```python
from build123d import *

# Parameters (mm, degrees)
SKETCH_1_W          = 30
SKETCH_1_H          = 30
EXTRUDE_1_DEPTH     = 7
SKETCH_2_W          = 8.25
SKETCH_2_H          = 8.25
CUT_EXTRUDE_1_DEPTH = 23.338307904
SKETCH_3_R          = 3
EXTRUDE_2_DEPTH     = 2
SKETCH_4_R          = 1.6
CUT_EXTRUDE_2_DEPTH = 5
SKETCH_5_R          = 12.625
CUT_EXTRUDE_3_DEPTH = 3
FILLET_1_R          = 15


with BuildPart() as part:
    # Эскиз1 → Бобышка-Вытянуть1 (new body)
    with BuildSketch(Plane.XY):
        Rectangle(SKETCH_1_W, SKETCH_1_H)
    extrude(amount=EXTRUDE_1_DEPTH)

    # Эскиз2 → Вырез-Вытянуть1 (cut, through all)
    with BuildSketch(Plane.XY.offset(7)):
        Rectangle(SKETCH_2_W, SKETCH_2_H)
    extrude(amount=-CUT_EXTRUDE_1_DEPTH, mode=Mode.SUBTRACT)

    # Эскиз3 → Бобышка-Вытянуть2 (add)
    with BuildSketch(Plane.XY.offset(7)):
        with Locations((11.5, 0)):
            Circle(SKETCH_3_R)
        with Locations(Location((-11.5, 0, 0), (0, 0, 180))):
            Circle(SKETCH_3_R)
    extrude(amount=EXTRUDE_2_DEPTH)

    # Эскиз4 → Вырез-Вытянуть2 (cut)
    with BuildSketch(Plane.XY.offset(9)):
        with Locations((-11.5, 0)):
            Circle(SKETCH_4_R)
        with Locations((11.5, 0)):
            Circle(SKETCH_4_R)
    extrude(amount=-CUT_EXTRUDE_2_DEPTH, mode=Mode.SUBTRACT)

    # Эскиз5 → Вырез-Вытянуть3 (cut)
    with BuildSketch(Plane(origin=(0, 0, 0), x_dir=(-1, 0, 0), z_dir=(0, 0, -1))):
        Circle(SKETCH_5_R)
    extrude(amount=-CUT_EXTRUDE_3_DEPTH, mode=Mode.SUBTRACT)

    # Скругление1
    fillet_1_edges = [part.edges().sort_by_distance(p)[0] for p in [
        (-15, 15, 3.5),
        (15, 15, 3.5),
        (15, -15, 3.5),
        (-15, -15, 3.5),
    ]]
    fillet(fillet_1_edges, radius=FILLET_1_R - 0.0001)  # a hair under: the kernel refuses the full size


solid = part.part
```
Geometry check sheet. Reference: the model listing, model coordinates, mm. A direction names the side the tool comes from. Coordinates: 2 decimals unless noted, no trailing zeros. Order: outer loops, then holes, each group sorted by start corner. A loop starts at its lowest first (then second) coordinate and runs counter-clockwise, first axis right, second up.
Q1. Depth check by flat-ended pin: pin 1 Ø1 at (x, y) = (10.5, -4) entering from -Z; pin 2 Ø1 at (y, z) = (-7.5, 2) entering from +X; pin 3 Ø1 at (x, z) = (6, 1.5) entering from +Y. Enter the tip coordinate at first touch or a pass-through.
Reply:
pin 1: stops at z = 3
pin 2: stops at x = 13.27
pin 3: stops at y = 13.96
Q2. Sectioned sample at D-D on x = 9.5. Record the cut outline in (y, z), and give its area (3 significant figures).
Reply:
outline: (-11.61, 0) - (-8.32, 0) - (-8.32, 3) - (8.32, 3) - (8.32, 0) - (11.61, 0) - (11.61, 7) - (2.24, 7) - (2.24, 9) - (-2.24, 9) - (-2.24, 7) - (-11.61, 7) - close
area: 122 mm2
Q3. Tool access check on faces 1 (the face through (0, 4.125, 5)), 2 (the face through (-10.72, 10.49, 3.55)), 3 (the face through (0, -5, 3)), 4 (the face through (-12, 0, 4)), 5 (the face through (10.49, -10.72, 3.55)). Record the directions out of +Z, -Z, +X, -X, +Y, -Y that give a thin tool (end or side, any length) a straight path to the whole face; none if there is none.
Reply:
face 1: +Z, -Z
face 2: +Z, -Z, -X, +Y
face 3: -Z
face 4: +Z
face 5: +Z, -Z, +X, -Y
Q4. Thickness scan on probe 1 along Y at (x, z) = (0, 2.2) (3 decimals); probe 2 along Z at (x, y) = (2, -4.5); probe 3 along X at (y, z) = (-2, 1). Record the ranges inside material, lowest first.
Reply:
probe 1: y = -15 to -12.625, 12.625 to 15
probe 2: z = 3 to 7
probe 3: x = -14.87 to -12.47, 12.47 to 14.87
Q5. Sectioned sample at B-B on z = 8.25. Record the cut outline in (x, y), and give its area (3 significant figures).
Reply:
outline: circle Ø6 at (-11.5, 0); circle Ø6 at (11.5, 0); hole circle Ø3.2 at (-11.5, 0); hole circle Ø3.2 at (11.5, 0)
area: 40.5 mm2
Q6. Draft check along Y on faces 6 (the face through (-8, -10, 0)), 7 (the face through (-8.5, -0.1, 8)), 8 (the face through (-4.125, 0, 5)). Enter one of: released by +Y, released by -Y, zero draft, split by the parting line, or undercut.
Reply:
face 6: zero draft
face 7: split by the parting line
face 8: undercut
Q7. Sectioned sample at C-C on x = 1.5. Record the cut outline in (y, z) (3 decimals).
Reply:
outline: (-14.925, 0) - (-12.536, 0) - (-12.536, 3) - (-4.125, 3) - (-4.125, 7) - (-14.925, 7) - close; (4.125, 3) - (12.536, 3) - (12.536, 0) - (14.925, 0) - (14.925, 7) - (4.125, 7) - close
